Design review of the part shown in the three views and the two pictorial views. Dimensions are in mm from the part's minimum x, y and z. Give positions to 0.01 mm unless a question says otherwise; leave off trailing zeros. Write each loop counter-clockwise with the first axis right and the second up, starting at its lowest first coordinate (ties: lowest second). Pieces come first, ordered by that corner, then holes. Notation, with made-up numbers: M 68.25,-38.5 L 100.25,-38.5 A5 cw 100.25,-29.5 Z; hole C 59.25,21 d7. An arc over 180 degrees is marked long. Write item = value, one per line.
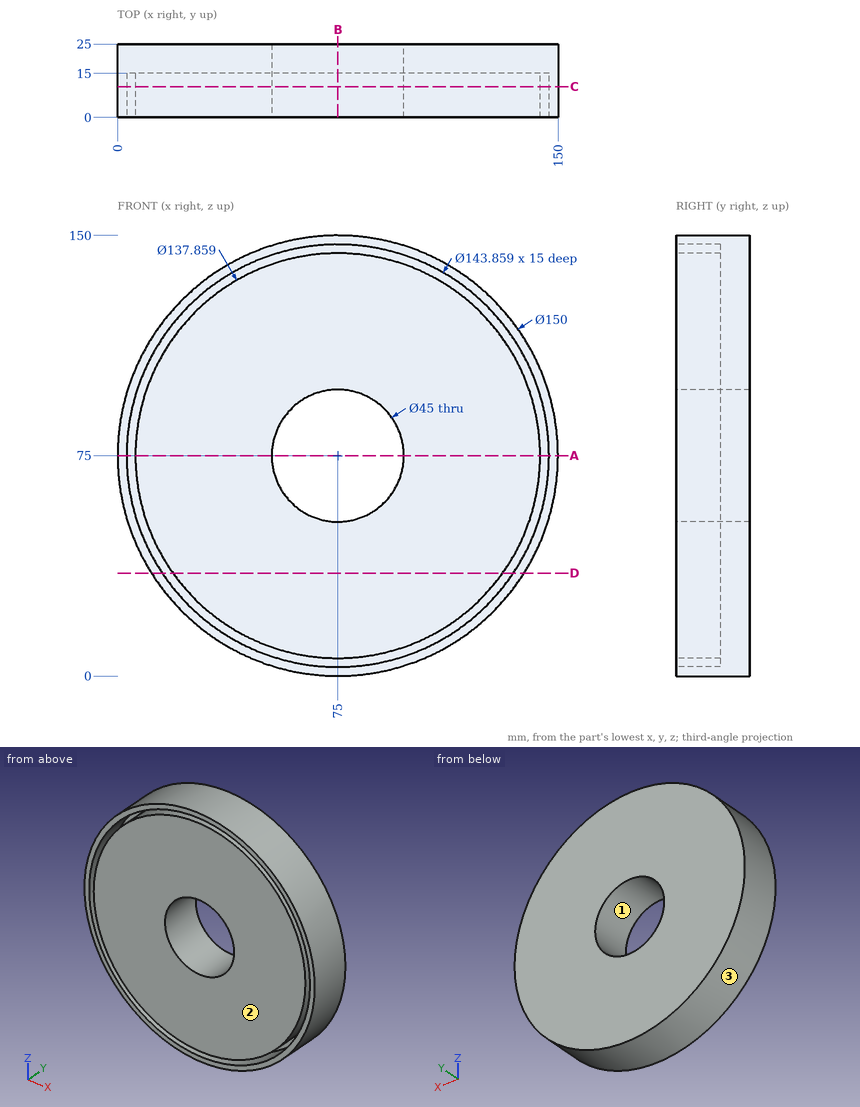
1. We need section A-A, the plane z = 75. Write out the cut boundary in (x, y), then the cut area to 4 significant figures.
Responses:
outline = M 0,0 L 3.07,0 L 3.07,15 L 6.07,15 L 6.07,0 L 52.5,0 L 52.5,25 L 0,25 Z; M 97.5,0 L 143.93,0 L 143.93,15 L 146.93,15 L 146.93,0 L 150,0 L 150,25 L 97.5,25 Z
area = 2,535 mm2
2. We need section D-D, the plane z = 35. Write out the cut boundary in (x, y), then the cut area to 3 significant figures.
Responses:
outline = M 11.56,0 L 15.22,0 L 15.22,15 L 18.86,15 L 18.86,0 L 131.14,0 L 131.14,15 L 134.78,15 L 134.78,0 L 138.44,0 L 138.44,25 L 11.56,25 Z
area = 3,060 mm2
3. Insertion check: P1, Ø6, axis at y = 16.5, z = 50.5, coming from the +X side; P2, Ø1, axis at x = 49, y = 8, coming from the +Z side; P3, Ø3, axis at x = 134.5, y = 12, coming from the -Z side. Each pin has a flat end and moves straight along its axis. Give the tip position at first contact, or say it passes through.
Responses:
P1 = 146.85
P2 = 145.53
P3 = 27.45
4. We need section B-B, the plane x = 75. Write out the cut boundary in (y, z), then the cut area to 4 significant figures.
Responses:
outline = M 0,0 L 25,0 L 25,52.5 L 0,52.5 L 0,6.07 L 15,6.07 L 15,3.07 L 0,3.07 Z; M 0,97.5 L 25,97.5 L 25,150 L 0,150 L 0,146.93 L 15,146.93 L 15,143.93 L 0,143.93 Z
area = 2,535 mm2
5. We need section C-C, the plane y = 10.5. Write out the cut boundary in (x, z).
Responses:
outline = C 75,75 d150; C 75,75 d137.86; hole C 75,75 d143.86; hole C 75,75 d45
6. The part is to be moulded in two halves that separate along Z. For the marked faces 1, 2 and 3, say which applies: +Z half, -Z half, draft (parallel to the pull), parting line (faces both ways), or undercut.
Responses:
face_1 = undercut
face_2 = draft
face_3 = parting line
7. For line 1 along Z through (x, y) = (75, 4); line 2 along Z through (x, y) = (61, 9) (1 decimal); line 3 along X through (y, z) = (1.5, 82.5) (1 decimal), list the stretches that pass through material, from the lowest coordinate up. Write a range as from..to.
Responses:
line_1 = 0..3.07, 6.07..52.5, 97.5..143.93, 146.93..150
line_2 = 1.3..4.4, 7.5..57.4, 92.6..142.5, 145.6..148.7
line_3 = 0.4..3.5, 6.5..53.8, 96.2..143.5, 146.5..149.6
